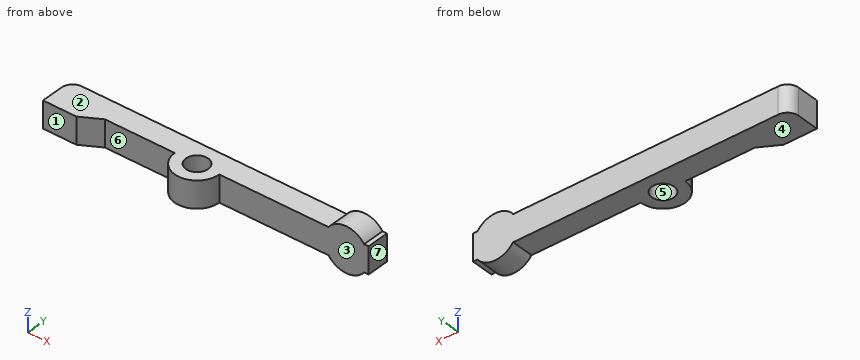
Autodesk Inventor part; units mm, degrees
ref_plane "YZ Plane" through (0, 0, 0) normal (1, 0, 0) x (0, 1, 0)
ref_plane "XZ Plane" through (0, 0, 0) normal (0, 1, 0) x (-1, 0, 0)
ref_plane "XY Plane" through (0, 0, 0) normal (0, 0, 1) x (1, 0, 0)
sketch "Esboço1" plane through (0, 0, 0) normal (0, 0, 1) x (1, 0, 0)
  arc A0 (-10, 0) -> (10, 0) centre (0, 0) ccw
  line L0 (10, 0) -> (77, 0)
  line L1 (77, 0) -> (77, 10)
  line L2 (77, 10) -> (-65, 10)
  line L3 (-65, 10) -> (-65, -5)
  line L4 (-65, -5) -> (-50, -5)
  line L5 (-50, -5) -> (-41.3397, 0)
  line L6 (-41.3397, 0) -> (-10, 0)
  dimension "d0" = 20
  dimension "d1" = 142
  dimension "d2" = 77
  dimension "d3" = 15
  dimension "d4" = 30
  dimension "d5" = 10
  dimension "d6" = 15
extrude "Extrusão1" add sketch "Esboço1" along normal mid plane 12
fillet "Arredondamento1" radius 5 1 edges at (-65, 10, 0)
sketch "Esboço2" plane through (0, 0, 6) normal (0, 0, 1) x (1, 0, 0)
  circle A0 centre (0, 0) radius 5
  dimension "d10" = 10
extrude "Extrusão2" cut sketch "Esboço2" against normal through all
sketch "Esboço3" plane through (77, 10, 6) normal (0, 1, 0) x (1, 0, 0)
  circle A0 centre (-10, 6) radius 10
  line L0 (0, 12) -> (0, 0)
  line L1 (-137, 0) -> (-137, 12)
  point P0 (-77, 6)
  point P1 (-137, 6)
  dimension "d13" = 20
  dimension "d14" = 10
extrude "Extrusão3" add sketch "Esboço3" against normal blind 10
properties material "Liga de aço"
Can you work these out from the model? Positions are in its coordinate system, mm. Face numbers are marked on the shaded views. A direction names the side the tool comes from. Give positions to 0.01 mm unless a question says otherwise; leave off trailing zeros. Order: outer loops, then holes, each group sorted by start corner. A loop starts at its lowest first (then second) coordinate and runs counter-clockwise, first axis right, second up. Notation, with made-up numbers: M 54,-8 L 106,-8 A23 ccw 106,12 Z; hole C 47,37.25 d5. An arc over 180 degrees is marked long. Use a Markdown table: item, result. Add a question column.
Item 1: We'd pull the mould along Y, two halves only. Please class the marked faces 5, 6 and 7: +Y half, -Y half, draft (parallel to the pull), parting line (faces both ways), or undercut.
Item 2: For the marked faces 1, 2, 3 and 4, which set-ups out of +Z, -Z, +X, -X, +Y, -Y let a thin tool reach every point of the face, with its end or its side?
Item 3: Suppose I cut it at D-D (y = 8.5). List the corners of the cut face in (x, z) for me, then the cut area to 3 significant figures.
Item 4: Suppose I cut it at C-C (y = 1.75). List the corners of the cut face in (x, z) for me, then the cut area to 3 significant figures.
Item 5: Suppose I cut it at B-B (z = -4.25). List the corners of the cut face in (x, y) for me.
Item 6: Suppose I cut it at A-A (x = 0). List the corners of the cut face in (y, z) for me, then the cut area to 3 significant figures.
Item 7: If I drill on L1, parallel to Y at x = 0, z = -3.5; L2, parallel to X at y = -0.75, z = -5.5; L3, parallel to Z at x = 36.5, y = 1.25, over which ranges is the centre line in solid material (lowest first)? Write a range as [from, to].
Item 8: Will these pins go through, and if not, where does the flat tip stop? pin 1 (1.6 mm diameter, centred on x = 76, y = 5.5, fed in from -Z); pin 2 (4 mm diameter, centred on x = 21.5, y = 3, fed in from +Z); pin 3 (3.5 mm diameter, centred on x = -60.5, z = 2.5, fed in from -Y); pin 4 (1.5 mm diameter, centred on y = 2.5, z = 6.5, fed in from +X).
Answer sheet:
| question | item | result |
|---|---|---|
| 1 | face 5 | undercut |
| 1 | face 6 | -Y half |
| 1 | face 7 | draft |
| 2 | face 1 | +Z, -Z, -X, -Y |
| 2 | face 2 | +Z, -X, +Y, -Y |
| 2 | face 3 | +Z, -Z, +X, -Y |
| 2 | face 4 | -Z, -X, +Y, -Y |
| 3 | outline | M -63.57,-6 L 59,-6 A10 ccw 75,-6 L 77,-6 L 77,6 L 75,6 A10 ccw 59,6 L -63.57,6 Z |
| 3 | area | 1,780 mm² |
| 4 | outline | M -65,-6 L -4.68,-6 L -4.68,6 L -65,6 Z; M 4.68,-6 L 59,-6 A10 ccw 75,-6 L 77,-6 L 77,6 L 75,6 A10 ccw 59,6 L 4.68,6 Z |
| 4 | area | 1,680 mm² |
| 5 | outline | M -65,-5 L -50,-5 L -41.34,0 L -10,0 A10 ccw 10,0 L 77,0 L 77,10 L -60,10 A5 ccw -65,5 Z; hole C 0,0 d10 |
| 6 | outline | M -10,-6 L -5,-6 L -5,6 L -10,6 Z; M 5,-6 L 10,-6 L 10,6 L 5,6 Z |
| 6 | area | 120 mm² |
| 7 | L1 | y = [-10, -5], [5, 10] |
| 7 | L2 | x = [-65, -42.64], [-9.97, -4.94], [4.94, 9.97] |
| 7 | L3 | z = [-6, 6] |
| 8 | pin 1 | stops at z = -6 |
| 8 | pin 2 | stops at z = 6 |
| 8 | pin 3 | stops at y = -5 |
| 8 | pin 4 | stops at x = 77 |
